```python
from build123d import *

# Parameters (mm, degrees)
SKETCH1_R           = 2.6035
BOSS_EXTRUDE1_DEPTH = 914.4
SKETCH2_W           = 573.8387108
SKETCH2_H           = 34.760821459
SKETCH2_W_2         = 1099.97900941
SKETCH2_H_2         = 36.169365112
CUT_EXTRUDE1_DEPTH  = 27.432


with BuildPart() as part:
    # Sketch1 → Boss-Extrude1 (new body, symmetric)
    with BuildSketch(Plane.XY):
        with BuildLine():
            Line((-7.179650497, -8.645192506), (-3.952270251, -5.423690499))
            ThreePointArc((-3.952270251, -5.423690499), (-2.922936451, -4.736929036), (-1.709253557, -4.4958))
            Line((-1.709253557, -4.4958), (1.709253557, -4.4958))
            ThreePointArc((1.709253557, -4.4958), (2.922936451, -4.736929036), (3.952270251, -5.423690499))
            Line((3.952270251, -5.423690499), (7.179650497, -8.645192506))
            ThreePointArc((7.179650497, -8.645192506), (7.41473083, -9.822813117), (6.416408329, -10.4902))
            Line((6.416408329, -10.4902), (4.287512407, -10.4902))
            ThreePointArc((4.287512407, -10.4902), (3.54574862, -10.79744862), (3.2385, -11.539212407))
            Line((3.2385, -11.539212407), (3.2385, -11.650987593))
            ThreePointArc((3.2385, -11.650987593), (3.54574862, -12.39275138), (4.287512407, -12.7))
            Line((4.287512407, -12.7), (5.317126718, -12.7))
            ThreePointArc((5.317126718, -12.7), (5.825126718, -12.192), (6.333126718, -12.7))
            Line((6.333126718, -12.7), (9.550443118, -12.7))
            ThreePointArc((9.550443118, -12.7), (10.058366869, -12.192000006), (10.566443095, -12.699847501))
            ThreePointArc((10.566443095, -12.699847501), (12.082537762, -12.08250727), (12.699846982, -10.566399977))
            ThreePointArc((12.699846982, -10.566399977), (12.192000006, -10.058323491), (12.7, -9.5504))
            Line((12.7, -9.5504), (12.7, -6.3330836))
            ThreePointArc((12.7, -6.3330836), (12.192, -5.8250836), (12.7, -5.3170836))
            Line((12.7, -5.3170836), (12.7, -4.287469289))
            ThreePointArc((12.7, -4.287469289), (12.39275138, -3.545705502), (11.650987593, -3.238456882))
            Line((11.650987593, -3.238456882), (11.539212407, -3.238456882))
            ThreePointArc((11.539212407, -3.238456882), (10.79744862, -3.545705502), (10.4902, -4.287469289))
            Line((10.4902, -4.287469289), (10.4902, -6.402089023))
            ThreePointArc((10.4902, -6.402089023), (9.856505071, -7.351067942), (8.737131347, -7.129408934))
            Line((8.737131347, -7.129408934), (5.441005833, -3.840816462))
            ThreePointArc((5.441005833, -3.840816462), (4.750877967, -2.809883091), (4.5085, -1.593185507))
            Line((4.5085, -1.593185507), (4.5085, 1.593185507))
            ThreePointArc((4.5085, 1.593185507), (4.750877967, 2.809883091), (5.441005833, 3.840816462))
            Line((5.441005833, 3.840816462), (8.737131347, 7.129408934))
            ThreePointArc((8.737131347, 7.129408934), (9.856505071, 7.351067942), (10.4902, 6.402089023))
            Line((10.4902, 6.402089023), (10.4902, 4.287469289))
            ThreePointArc((10.4902, 4.287469289), (10.79744862, 3.545705502), (11.539212407, 3.238456882))
            Line((11.539212407, 3.238456882), (11.650987593, 3.238456882))
            ThreePointArc((11.650987593, 3.238456882), (12.39275138, 3.545705502), (12.7, 4.287469289))
            Line((12.7, 4.287469289), (12.7, 5.3170836))
            ThreePointArc((12.7, 5.3170836), (12.192, 5.8250836), (12.7, 6.3330836))
            Line((12.7, 6.3330836), (12.7, 9.5504))
            ThreePointArc((12.7, 9.5504), (12.192000006, 10.058323491), (12.699846982, 10.566399977))
            ThreePointArc((12.699846982, 10.566399977), (12.082537762, 12.08250727), (10.566443095, 12.699847501))
            ThreePointArc((10.566443095, 12.699847501), (10.058366869, 12.192000006), (9.550443118, 12.7))
            Line((9.550443118, 12.7), (6.333126718, 12.7))
            ThreePointArc((6.333126718, 12.7), (5.825126718, 12.192), (5.317126718, 12.7))
            Line((5.317126718, 12.7), (4.287512407, 12.7))
            ThreePointArc((4.287512407, 12.7), (3.54574862, 12.39275138), (3.2385, 11.650987593))
            Line((3.2385, 11.650987593), (3.2385, 11.539212407))
            ThreePointArc((3.2385, 11.539212407), (3.54574862, 10.79744862), (4.287512407, 10.4902))
            Line((4.287512407, 10.4902), (6.476788598, 10.4902))
            ThreePointArc((6.476788598, 10.4902), (7.432222385, 9.85140422), (7.207036008, 8.724370562))
            Line((7.207036008, 8.724370562), (3.898272566, 5.423169045))
            ThreePointArc((3.898272566, 5.423169045), (2.869120213, 4.736787962), (1.655778399, 4.4958))
            Line((1.655778399, 4.4958), (-1.655778399, 4.4958))
            ThreePointArc((-1.655778399, 4.4958), (-2.869120213, 4.736787962), (-3.898272566, 5.423169045))
            Line((-3.898272566, 5.423169045), (-7.207036008, 8.724370562))
            ThreePointArc((-7.207036008, 8.724370562), (-7.432222385, 9.85140422), (-6.476788598, 10.4902))
            Line((-6.476788598, 10.4902), (-4.287512407, 10.4902))
            ThreePointArc((-4.287512407, 10.4902), (-3.54574862, 10.79744862), (-3.2385, 11.539212407))
            Line((-3.2385, 11.539212407), (-3.2385, 11.650987593))
            ThreePointArc((-3.2385, 11.650987593), (-3.54574862, 12.39275138), (-4.287512407, 12.7))
            Line((-4.287512407, 12.7), (-5.317126718, 12.7))
            ThreePointArc((-5.317126718, 12.7), (-5.825126718, 12.192), (-6.333126718, 12.7))
            Line((-6.333126718, 12.7), (-9.550443118, 12.7))
            ThreePointArc((-9.550443118, 12.7), (-10.058366869, 12.192000006), (-10.566443095, 12.699847501))
            ThreePointArc((-10.566443095, 12.699847501), (-12.082537762, 12.08250727), (-12.699846982, 10.566399977))
            ThreePointArc((-12.699846982, 10.566399977), (-12.192000006, 10.058323491), (-12.7, 9.5504))
            Line((-12.7, 9.5504), (-12.7, 6.3330836))
            ThreePointArc((-12.7, 6.3330836), (-12.192, 5.8250836), (-12.7, 5.3170836))
            Line((-12.7, 5.3170836), (-12.7, 4.287469289))
            ThreePointArc((-12.7, 4.287469289), (-12.39275138, 3.545705502), (-11.650987593, 3.238456882))
            Line((-11.650987593, 3.238456882), (-11.539212407, 3.238456882))
            ThreePointArc((-11.539212407, 3.238456882), (-10.79744862, 3.545705502), (-10.4902, 4.287469289))
            Line((-10.4902, 4.287469289), (-10.4902, 6.402089023))
            ThreePointArc((-10.4902, 6.402089023), (-9.856505071, 7.351067942), (-8.737131347, 7.129408934))
            Line((-8.737131347, 7.129408934), (-5.441005833, 3.840816462))
            ThreePointArc((-5.441005833, 3.840816462), (-4.750877967, 2.809883091), (-4.5085, 1.593185507))
            Line((-4.5085, 1.593185507), (-4.5085, -1.593185507))
            ThreePointArc((-4.5085, -1.593185507), (-4.750877967, -2.809883091), (-5.441005833, -3.840816462))
            Line((-5.441005833, -3.840816462), (-8.737131347, -7.129408934))
            ThreePointArc((-8.737131347, -7.129408934), (-9.856505071, -7.351067942), (-10.4902, -6.402089023))
            Line((-10.4902, -6.402089023), (-10.4902, -4.287469289))
            ThreePointArc((-10.4902, -4.287469289), (-10.79744862, -3.545705502), (-11.539212407, -3.238456882))
            Line((-11.539212407, -3.238456882), (-11.650987593, -3.238456882))
            ThreePointArc((-11.650987593, -3.238456882), (-12.39275138, -3.545705502), (-12.7, -4.287469289))
            Line((-12.7, -4.287469289), (-12.7, -5.3170836))
            ThreePointArc((-12.7, -5.3170836), (-12.192, -5.8250836), (-12.7, -6.3330836))
            Line((-12.7, -6.3330836), (-12.7, -9.5504))
            ThreePointArc((-12.7, -9.5504), (-12.192000006, -10.058323491), (-12.699846982, -10.566399977))
            ThreePointArc((-12.699846982, -10.566399977), (-12.082537762, -12.08250727), (-10.566443095, -12.699847501))
            ThreePointArc((-10.566443095, -12.699847501), (-10.058366869, -12.192000006), (-9.550443118, -12.7))
            Line((-9.550443118, -12.7), (-6.333126718, -12.7))
            ThreePointArc((-6.333126718, -12.7), (-5.825126718, -12.192), (-5.317126718, -12.7))
            Line((-5.317126718, -12.7), (-4.287512407, -12.7))
            ThreePointArc((-4.287512407, -12.7), (-3.54574862, -12.39275138), (-3.2385, -11.650987593))
            Line((-3.2385, -11.650987593), (-3.2385, -11.539212407))
            ThreePointArc((-3.2385, -11.539212407), (-3.54574862, -10.79744862), (-4.287512407, -10.4902))
            Line((-4.287512407, -10.4902), (-6.416408329, -10.4902))
            ThreePointArc((-6.416408329, -10.4902), (-7.41473083, -9.822813117), (-7.179650497, -8.645192506))
        make_face()
        Circle(SKETCH1_R, mode=Mode.SUBTRACT)
    extrude(amount=BOSS_EXTRUDE1_DEPTH, both=True)

    # Sketch2 → Cut-Extrude1 (cut)
    with BuildSketch(Plane(origin=(12.7, 0, 0), x_dir=(0, 0, -1), z_dir=(1, 0, 0))):
        with Locations((-631.537917207, -0.58573738)):
            Rectangle(SKETCH2_W, SKETCH2_H)
        with Locations((375.067711741, 0.118534447)):
            Rectangle(SKETCH2_W_2, SKETCH2_H_2)
    extrude(amount=-CUT_EXTRUDE1_DEPTH, mode=Mode.SUBTRACT)


solid = part.part
```
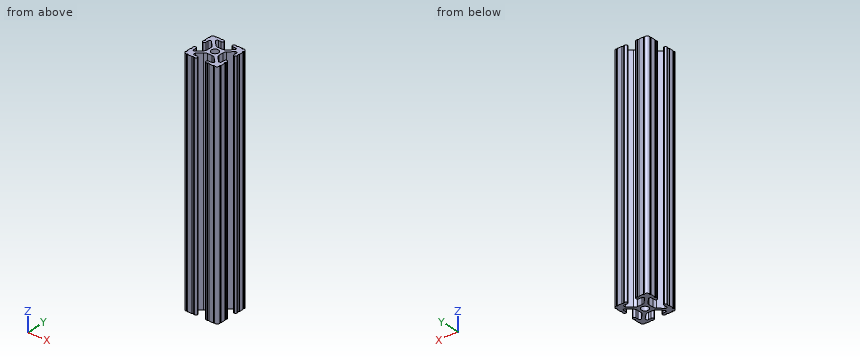
Model file for the job. Use its own axes, mm. Give positions to 0.01 mm unless a question says otherwise; leave off trailing zeros. Write each loop counter-clockwise with the first axis right and the second up, starting at its lowest first coordinate (ties: lowest second). Pieces come first, ordered by that corner, then holes. Notation, with made-up numbers: (13.5, 83.5) -> (60.5, 83.5) arc R22 ccw to (60.5, 111.5) -> close; hole circle Ø11 at (66, 42). An arc over 180 degrees is marked (long way). Use CSV: the item, a comma, the result in double quotes. Start each with the question number.
1) Cut at A-A on y = 0. List the corners of the cut face in (x, z), plus the area to 3 significant figures.
2) Cut at B-B on x = 0. List the corners of the cut face in (y, z), plus the area to 3 significant figures.
3) Drill centre lines: L1, parallel to X at y = 0, z = 259.5; L2, parallel to Y at x = 0, z = 310.5; L3, parallel to X at y = 3.5, z = 275. Where is each one in solid material? Low to high.
4) Pin check, flat tips, straight feed: P1, Ø1.7, axis at x = -0.5, z = 262, coming from the +Y side; P2, Ø1, axis at y = 0, z = 256.5, coming from the -X side; P3, Ø4, axis at y = 1, z = 212, coming from the -X side. Stop position of each tip, or through.
Final values:
1,outline,"(-4.51, 174.92) -> (-2.6, 174.92) -> (-2.6, 344.62) -> (-4.51, 344.62) -> close; (2.6, 174.92) -> (4.51, 174.92) -> (4.51, 344.62) -> (2.6, 344.62) -> close"
1,area,"647 mm2"
2,outline,"(-4.5, 174.92) -> (-2.6, 174.92) -> (-2.6, 344.62) -> (-4.5, 344.62) -> close; (2.6, 174.92) -> (4.5, 174.92) -> (4.5, 344.62) -> (2.6, 344.62) -> close"
2,area,"642 mm2"
3,L1,"x = -4.51 to -2.6, 2.6 to 4.51"
3,L2,"y = -4.5 to -2.6, 2.6 to 4.5"
3,L3,"x = -12.34 to -10.85, -5.14 to 5.14, 10.85 to 12.34"
4,P1,"stops at y = 4.5"
4,P2,"stops at x = -4.51"
4,P3,"stops at x = -4.84"
